from build123d import *

# Parameters (mm, degrees)
SKETCH1_R           = 110
SKETCH1_W           = 20
SKETCH1_H           = 5
SKETCH1_W_2         = 5
SKETCH1_H_2         = 30
BOSS_EXTRUDE1_DEPTH = 5


with BuildPart() as part:
    # Sketch1 → Boss-Extrude1 (new body)
    with BuildSketch(Plane.XY):
        Circle(SKETCH1_R)
        with Locations((-20, 57.5)):
            Rectangle(SKETCH1_W, SKETCH1_H, mode=Mode.SUBTRACT)
        with Locations((20, 57.5)):
            Rectangle(SKETCH1_W, SKETCH1_H, mode=Mode.SUBTRACT)
        with Locations((37.5, 35)):
            Rectangle(SKETCH1_W_2, SKETCH1_H_2, mode=Mode.SUBTRACT)
        with Locations((37.5, -35)):
            Rectangle(SKETCH1_W_2, SKETCH1_H_2, mode=Mode.SUBTRACT)
        with Locations((20, -57.5)):
            Rectangle(SKETCH1_W, SKETCH1_H, mode=Mode.SUBTRACT)
        with Locations((-20, -57.5)):
            Rectangle(SKETCH1_W, SKETCH1_H, mode=Mode.SUBTRACT)
        with Locations((-37.5, -35)):
            Rectangle(SKETCH1_W_2, SKETCH1_H_2, mode=Mode.SUBTRACT)
        with Locations((-37.5, 35)):
            Rectangle(SKETCH1_W_2, SKETCH1_H_2, mode=Mode.SUBTRACT)
    extrude(amount=BOSS_EXTRUDE1_DEPTH)


solid = part.part
For this review, take the finished solid that the model builds, in its own axes (mm). Round coordinates to 2 decimals unless told otherwise and drop trailing zeros. Loops run counter-clockwise (first coordinate to the right, second up) from the corner with the lowest first, then second, coordinate; pieces in that order, holes last. Notation, with made-up numbers: (-32, 49.25) - (24, 49.25) arc R11 cw to (24, 66.25) - close; hole circle Ø3 at (-22, -40). An arc over 180 degrees is marked (long way). Answer as CSV lines item,"result".
(1) Consider section D-D on x = -71. Give the boundary of the cut face in (y, z), then the cut area to 3 significant figures.
Checked values:
outline,"(-84.02, 0) - (84.02, 0) - (84.02, 5) - (-84.02, 5) - close"
area,"840 mm2"
(2) Consider section C-C on y = -27. Give the boundary of the cut face in (x, z).
Checked values:
outline,"(-106.63, 0) - (-40, 0) - (-40, 5) - (-106.63, 5) - close; (-35, 0) - (35, 0) - (35, 5) - (-35, 5) - close; (40, 0) - (106.63, 0) - (106.63, 5) - (40, 5) - close"
(3) Mouldability with a two-part tool opening along X and no side actions: class faces 1 (the face through (-38, -50, 2)), 2 (the face through (-2, 2, 5)), 3 (the face through (-23.846, -107.384, 2.465)), 4 (the face through (35, -35, 2)) as +X half, -X half, draft (parallel to the pull), parting line (faces both ways), or undercut.
Checked values:
face 1,"undercut"
face 2,"draft"
face 3,"parting line"
face 4,"undercut"
(4) Insertion check: P1, Ø5, axis at x = 78, y = -65.5, coming from the -Z side; P2, Ø1.5, axis at x = 22.5, z = 2, coming from the +Y side; P3, Ø2.5, axis at y = -32.5, z = 3.5, coming from the +X side; P4, Ø1.5, axis at x = -37, z = 2.5, coming from the -Y side. Each pin has a flat end and moves straight along its axis. Give the tip position at first contact, or say it passes through.
Checked values:
P1,"stops at z = 0"
P2,"stops at y = 107.83"
P3,"stops at x = 105.47"
P4,"stops at y = -103.86"
(5) Consider section A-A on y = 24. Give the boundary of the cut face in (x, z).
Checked values:
outline,"(-107.35, 0) - (-40, 0) - (-40, 5) - (-107.35, 5) - close; (-35, 0) - (35, 0) - (35, 5) - (-35, 5) - close; (40, 0) - (107.35, 0) - (107.35, 5) - (40, 5) - close"
(6) Wall thickness on line 1 (X direction, y = -46.5, z = 4.6); line 2 (X direction, y = -21, z = 4.5); line 3 (Y direction, x = 19.5, z = 3.95): over which ranges is each line inside the solid? List them lowest first.
Checked values:
line 1,"x = -99.69 to -40, -35 to 35, 40 to 99.69"
line 2,"x = -107.98 to -40, -35 to 35, 40 to 107.98"
line 3,"y = -108.26 to -60, -55 to 55, 60 to 108.26"
(7) Consider section B-B on z = 1.75. Give the number of separate pieces and of enclosed holes in the cut face, then the cut area to 3 significant figures.
Checked values:
separate pieces,"1"
enclosed holes,"8"
area,"37,000 mm2"
